from build123d import *

# Parameters (mm, degrees)
F2_SIZE = 0.35


with BuildPart() as f1:
    # F0 (on Front) → F1 (revolve)
    with BuildSketch(Plane.XZ):
        Polygon((0, 1.65), (0, 3), (-2, 3), (-2, 4), (-22, 4), (-22, 3), (-24, 3), (-24, 1.65), align=None)
    revolve(axis=Axis((-12, 0, 0), (-1, 0, 0)))

    # F2
    f2_edges = [f1.edges().sort_by_distance(p)[0] for p in [
        (-24, 0, -1.65),
        (0, 0, -1.65),
    ]]
    chamfer(f2_edges, length=F2_SIZE)


solid = f1.part
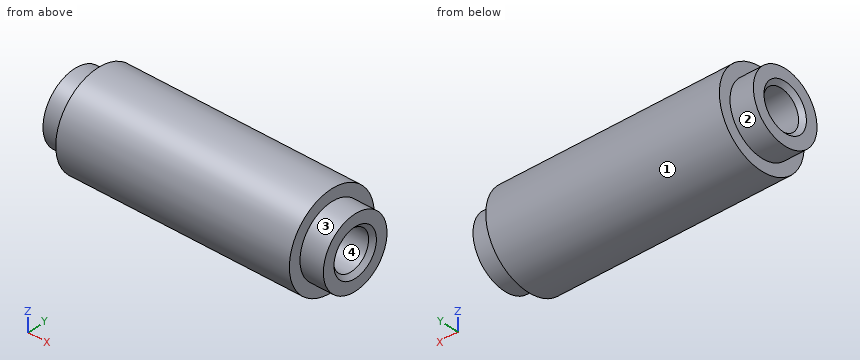
Can you work these out from the model? Positions are in its coordinate system, mm. Face numbers are marked on the shaded views. A direction names the side the tool comes from. Round coordinates to 2 decimals unless told otherwise and drop trailing zeros. Loops run counter-clockwise (first coordinate to the right, second up) from the corner with the lowest first, then second, coordinate; pieces in that order, holes last. Notation, with made-up numbers: (52, 0.25) - (81, 0.25) arc R16 cw to (81, 24.25) - close; hole circle Ø3 at (5.25, 55). An arc over 180 degrees is marked (long way). Answer in a Markdown table with one row per item. Add a question column.
Q1. I need wall thicknesses on L1, parallel to Y at x = -17, z = 0; L2, parallel to X at y = -2.5, z = -2.5; L3, parallel to Z at x = -14.5, y = -0.5. Which ranges of each line are inside material? Lowest first, please.
Q2. I want a section at D-D on z = -2.25. List the corners of the cut face in (x, y) for me, and give its area (3 significant figures).
Q3. We'd pull the mould along Z, two halves only. Please class the marked faces 3 and 4: pulls with the +Z half, pulls with the -Z half, needs draft (parallel to the pull), parting line crosses it, or undercut.
Q4. I want a section at A-A on z = 0. List the corners of the cut face in (x, y) for me.
Q5. Which directions (+Z, -Z, +X, -X, +Y, -Y) give clear straight access to the entire face, cutting with the end or side of a thin tool? Please do the marked faces 1 and 2.
Q6. I want a section at C-C on x = -18. List the corners of the cut face in (y, z) for me.
Q7. For pin 1 Ø1.5 at (x, z) = (-2.5, -2) entering from -Y; pin 2 Ø2.5 at (y, z) = (0, 0.5) entering from +X, each with a flat end and sliding along its axis, tell me the tip position at first contact or that it passes through.
A:
| question | item | result |
|---|---|---|
| 1 | L1 | -4 to -1.65, 1.65 to 4 |
| 1 | L2 | -22 to -2 |
| 1 | L3 | -3.97 to -1.57, 1.57 to 3.97 |
| 2 | outline | (-24, -1.98) - (-22, -1.98) - (-22, -3.31) - (-2, -3.31) - (-2, -1.98) - (0, -1.98) - (0, 1.98) - (-2, 1.98) - (-2, 3.31) - (-22, 3.31) - (-22, 1.98) - (-24, 1.98) - close |
| 2 | area | 148 mm^2 |
| 3 | face 3 | parting line crosses it |
| 3 | face 4 | undercut |
| 4 | outline | (-24, -3) - (-22, -3) - (-22, -4) - (-2, -4) - (-2, -3) - (0, -3) - (0, -2) - (-0.35, -1.65) - (-23.65, -1.65) - (-24, -2) - close; (-24, 2) - (-23.65, 1.65) - (-0.35, 1.65) - (0, 2) - (0, 3) - (-2, 3) - (-2, 4) - (-22, 4) - (-22, 3) - (-24, 3) - close |
| 5 | face 1 | +X, -X |
| 5 | face 2 | -X |
| 6 | outline | circle Ø8 at (0, 0); hole circle Ø3.3 at (0, 0) |
| 7 | pin 1 | y = -3.8 |
| 7 | pin 2 | x = -0.25 |
